from build123d import *

# Parameters (mm, degrees)
SKETCH1_R           = 2.8625
BOSS_EXTRUDE1_DEPTH = 5
SKETCH2_R           = 2.8625
SKETCH2_R_2         = 1.46
BOSS_EXTRUDE2_DEPTH = 1


with BuildPart() as part:
    # Sketch1 → Boss-Extrude1 (new body)
    with BuildSketch(Plane(origin=(0, 0, 0), x_dir=(1, 0, 0), z_dir=(0, 1, 0))):
        with BuildLine():
            Line((-0.575, 7.126841867), (0, 7.126841867))
            Line((0, 7.126841867), (0.575, 7.126841867))
            ThreePointArc((0.575, 7.126841867), (0.941802699, 6.263909422), (0.875, 5.328637255))
            ThreePointArc((0.875, 5.328637255), (0.903794388, 4.983429203), (1.167554815, 4.758867066))
            Line((1.167554815, 4.758867066), (1.852620192, 4.536275832))
            ThreePointArc((1.852620192, 4.536275832), (2.198001172, 4.562915928), (2.424204523, 4.825270192))
            ThreePointArc((2.424204523, 4.825270192), (2.919899191, 5.62118691), (3.723867773, 6.103712707))
            Line((3.723867773, 6.103712707), (4.189052545, 5.765736187))
            Line((4.189052545, 5.765736187), (4.654237317, 5.427759667))
            ThreePointArc((4.654237317, 5.427759667), (4.443767969, 4.514031436), (3.839984264, 3.796646001))
            ThreePointArc((3.839984264, 3.796646001), (3.660371211, 3.500441903), (3.741763566, 3.163732829))
            Line((3.741763566, 3.163732829), (4.165157254, 2.580981412))
            ThreePointArc((4.165157254, 2.580981412), (4.460234992, 2.399523856), (4.797445315, 2.478813921))
            ThreePointArc((4.797445315, 2.478813921), (5.666298834, 2.831362057), (6.600344627, 2.74917275))
            Line((6.600344627, 2.74917275), (6.778029398, 2.202315253))
            Line((6.778029398, 2.202315253), (6.95571417, 1.655457756))
            ThreePointArc((6.95571417, 1.655457756), (6.248364912, 1.039946868), (5.338225055, 0.814465017))
            ThreePointArc((5.338225055, 0.814465017), (5.018810642, 0.680404772), (4.886745813, 0.360160182))
            Line((4.886745813, 0.360160182), (4.886745813, -0.360160182))
            ThreePointArc((4.886745813, -0.360160182), (5.018810642, -0.680404772), (5.338225055, -0.814465017))
            ThreePointArc((5.338225055, -0.814465017), (6.248364912, -1.039946868), (6.95571417, -1.655457756))
            Line((6.95571417, -1.655457756), (6.778029398, -2.202315253))
            Line((6.778029398, -2.202315253), (6.600344627, -2.74917275))
            ThreePointArc((6.600344627, -2.74917275), (5.666298834, -2.831362057), (4.797445315, -2.478813921))
            ThreePointArc((4.797445315, -2.478813921), (4.460234992, -2.399523856), (4.165157254, -2.580981412))
            Line((4.165157254, -2.580981412), (3.741763566, -3.163732829))
            ThreePointArc((3.741763566, -3.163732829), (3.660371211, -3.500441903), (3.839984264, -3.796646001))
            ThreePointArc((3.839984264, -3.796646001), (4.443767969, -4.514031436), (4.654237317, -5.427759667))
            Line((4.654237317, -5.427759667), (4.189052545, -5.765736187))
            Line((4.189052545, -5.765736187), (3.723867773, -6.103712707))
            ThreePointArc((3.723867773, -6.103712707), (2.919899191, -5.62118691), (2.424204523, -4.825270192))
            ThreePointArc((2.424204523, -4.825270192), (2.198001172, -4.562915928), (1.852620192, -4.536275832))
            Line((1.852620192, -4.536275832), (1.167554815, -4.758867066))
            ThreePointArc((1.167554815, -4.758867066), (0.903794388, -4.983429203), (0.875, -5.328637255))
            ThreePointArc((0.875, -5.328637255), (0.941802699, -6.263909422), (0.575, -7.126841867))
            Line((0.575, -7.126841867), (0, -7.126841867))
            Line((0, -7.126841867), (-0.575, -7.126841867))
            ThreePointArc((-0.575, -7.126841867), (-0.941802699, -6.263909422), (-0.875, -5.328637255))
            ThreePointArc((-0.875, -5.328637255), (-0.903794388, -4.983429203), (-1.167554815, -4.758867066))
            Line((-1.167554815, -4.758867066), (-1.852620192, -4.536275832))
            ThreePointArc((-1.852620192, -4.536275832), (-2.198001172, -4.562915928), (-2.424204523, -4.825270192))
            ThreePointArc((-2.424204523, -4.825270192), (-2.919899191, -5.62118691), (-3.723867773, -6.103712707))
            Line((-3.723867773, -6.103712707), (-4.189052545, -5.765736187))
            Line((-4.189052545, -5.765736187), (-4.654237317, -5.427759667))
            ThreePointArc((-4.654237317, -5.427759667), (-4.443767969, -4.514031436), (-3.839984264, -3.796646001))
            ThreePointArc((-3.839984264, -3.796646001), (-3.660371211, -3.500441903), (-3.741763566, -3.163732829))
            Line((-3.741763566, -3.163732829), (-4.165157254, -2.580981412))
            ThreePointArc((-4.165157254, -2.580981412), (-4.460234992, -2.399523856), (-4.797445315, -2.478813921))
            ThreePointArc((-4.797445315, -2.478813921), (-5.666298834, -2.831362057), (-6.600344627, -2.74917275))
            Line((-6.600344627, -2.74917275), (-6.778029398, -2.202315253))
            Line((-6.778029398, -2.202315253), (-6.95571417, -1.655457756))
            ThreePointArc((-6.95571417, -1.655457756), (-6.248364912, -1.039946868), (-5.338225055, -0.814465017))
            ThreePointArc((-5.338225055, -0.814465017), (-5.018810642, -0.680404772), (-4.886745813, -0.360160182))
            Line((-4.886745813, -0.360160182), (-4.886745813, 0.360160182))
            ThreePointArc((-4.886745813, 0.360160182), (-5.018810642, 0.680404772), (-5.338225055, 0.814465017))
            ThreePointArc((-5.338225055, 0.814465017), (-6.248364912, 1.039946868), (-6.95571417, 1.655457756))
            Line((-6.95571417, 1.655457756), (-6.778029398, 2.202315253))
            Line((-6.778029398, 2.202315253), (-6.600344627, 2.74917275))
            ThreePointArc((-6.600344627, 2.74917275), (-5.666298834, 2.831362057), (-4.797445315, 2.478813921))
            ThreePointArc((-4.797445315, 2.478813921), (-4.460234992, 2.399523856), (-4.165157254, 2.580981412))
            Line((-4.165157254, 2.580981412), (-3.741763566, 3.163732829))
            ThreePointArc((-3.741763566, 3.163732829), (-3.660371211, 3.500441903), (-3.839984264, 3.796646001))
            ThreePointArc((-3.839984264, 3.796646001), (-4.443767969, 4.514031436), (-4.654237317, 5.427759667))
            Line((-4.654237317, 5.427759667), (-4.189052545, 5.765736187))
            Line((-4.189052545, 5.765736187), (-3.723867773, 6.103712707))
            ThreePointArc((-3.723867773, 6.103712707), (-2.919899191, 5.62118691), (-2.424204523, 4.825270192))
            ThreePointArc((-2.424204523, 4.825270192), (-2.198001172, 4.562915928), (-1.852620192, 4.536275832))
            Line((-1.852620192, 4.536275832), (-1.167554815, 4.758867066))
            ThreePointArc((-1.167554815, 4.758867066), (-0.903794388, 4.983429203), (-0.875, 5.328637255))
            ThreePointArc((-0.875, 5.328637255), (-0.941802699, 6.263909422), (-0.575, 7.126841867))
        make_face()
        with Locations(Location((0, 0, 0), (0, 0, 270))):
            Circle(SKETCH1_R, mode=Mode.SUBTRACT)
    extrude(amount=BOSS_EXTRUDE1_DEPTH)

    # Sketch2 → Boss-Extrude2 (add)
    with BuildSketch(Plane(origin=(0, 4, 0), x_dir=(1, 0, 0), z_dir=(0, 1, 0))):
        with Locations(Location((0, 0, 0), (0, 0, 270))):
            Circle(SKETCH2_R)
        with Locations(Location((0, 0, 0), (0, 0, 270))):
            Circle(SKETCH2_R_2, mode=Mode.SUBTRACT)
    extrude(amount=BOSS_EXTRUDE2_DEPTH)


solid = part.part
Design review of the part built by this model. Coordinates are the model's own, in mm. A direction names the side the tool comes from. Give positions to 0.01 mm unless a question says otherwise; leave off trailing zeros. Order: outer loops, then holes, each group sorted by start corner. A loop starts at its lowest first (then second) coordinate and runs counter-clockwise, first axis right, second up. Notation, with made-up numbers: (54, -26) - (102, -26) arc R28 cw to (102, -3) - close; hole circle Ø1 at (-28.75, 79). An arc over 180 degrees is marked (long way). Use CSV: the item, a comma, the result in double quotes. Start each with the question number.
Q1. Take a section at A-A (z = 0). State the section outline as (x, y) points.
Q2. Take a section at B-B (x = 0). State the section outline as (y, z) points.
Q3. For P1, Ø3, axis at x = 5.5, y = 1, coming from the -Z side; P2, Ø0.6, axis at y = 3.5, z = 0, coming from the -X side; P3, Ø1.5, axis at x = 4, y = 2, coming from the +Z side, all flat-tipped, find the tip position at first contact; note any pin that passes through.
Q4. For line 1 (Z direction, x = 3.75, y = 4.1); line 2 (X direction, y = 3.85, z = 5.75); line 3 (Z direction, x = 4.25, y = 4.6), list the stretches that pass through material, from the lowest coordinate up.
Q5. Draft analysis for pull direction Z (two halves, no side actions). For faces 1 (the face through (5.679, 2.465, 2.833)), 2 (the face through (4.45, 2.46, -4.53)), 3 (the face through (0, 2, -7.127)), 4 (the face through (4.438, 2.465, 4.502)), state which applies: pulls with the +Z half, pulls with the -Z half, needs draft (parallel to the pull), parting line crosses it, or undercut.
Q6. Take a section at C-C (z = 4). State the section outline as (x, y) points, and give its area (3 significant figures).
Q7. Machinability: for faces 5 (the face through (2.9, 2.5, 5.6)), 6 (the face through (-2.9, 2.5, -5.6)), 7 (the face through (-2.8, 2, -0.6)), 8 (the face through (-0.94, 2.46, 6.28)), which of the approach directions +Z, -Z, +X, -X, +Y, -Y give a long, thin tool a straight path to every point of the face, cutting with its end or side? Answer none if there is none.
Calculated:
1,outline,"(-4.89, 0) - (-2.86, 0) - (-2.86, 4) - (-1.46, 4) - (-1.46, 5) - (-4.89, 5) - close; (1.46, 4) - (2.86, 4) - (2.86, 0) - (4.89, 0) - (4.89, 5) - (1.46, 5) - close"
2,outline,"(0, -7.13) - (5, -7.13) - (5, -1.46) - (4, -1.46) - (4, -2.86) - (0, -2.86) - close; (0, 2.86) - (4, 2.86) - (4, 1.46) - (5, 1.46) - (5, 7.13) - (0, 7.13) - close"
3,P1,"stops at z = -5.9"
3,P2,"stops at x = -4.89"
3,P3,"stops at z = 6.1"
4,line 1,"z = -6.08 to -3.71, -3.15 to 3.15, 3.71 to 6.08"
4,line 2,"x = -4.21 to -3.06, -0.96 to 0.96, 3.06 to 4.21"
4,line 3,"z = -5.72 to -4.2, -2.49 to 2.49, 4.2 to 5.72"
5,face 1,"pulls with the +Z half"
5,face 2,"undercut"
5,face 3,"pulls with the -Z half"
5,face 4,"undercut"
6,outline,"(-4.08, 0) - (4.08, 0) - (4.08, 5) - (-4.08, 5) - close"
6,area,"40.8 mm²"
7,face 5,"+Z, +Y, -Y"
7,face 6,"-Z, +Y, -Y"
7,face 7,"-Y"
7,face 8,"+Y, -Y"
